```python
from build123d import *

# Parameters (mm, degrees)
F0_R     = 2.0574
F1_DEPTH = 12.7


# Not quite as in the source:
# - a feature names something its author has since deleted; it is built from what else it names


with BuildPart() as f1:
    # F0 (on Top) → F1 (new body)
    with BuildSketch(Plane.XY):
        with BuildLine():
            Line((0, 8.9704120984), (0, -13.0232248562))
            Line((0, -13.0232248562), (26.7917899333, -13.0232248562))
            ThreePointArc((26.7917899333, -13.0232248562), (29.7688, -0.5781617802), (32.7458100667, -13.0232248562))
            Line((32.7458100667, -13.0232248562), (59.5376, -13.0232248562))
            Line((59.5376, -13.0232248562), (59.5376, 8.9704120984))
            Line((59.5376, 8.9704120984), (0, 8.9704120984))
        make_face()
        with Locations((8.1026, -5.2786845261)):
            Circle(F0_R, mode=Mode.SUBTRACT)
        with Locations((51.435, -5.2786845261)):
            Circle(F0_R, mode=Mode.SUBTRACT)
    extrude(amount=F1_DEPTH)


solid = f1.part
```
Check sheet for the modelled part. Datum: model origin and axes. Units: mm. Round coordinates to 2 decimals unless told otherwise and drop trailing zeros. Loops run counter-clockwise (first coordinate to the right, second up) from the corner with the lowest first, then second, coordinate; pieces in that order, holes last. Notation, with made-up numbers: (89, -13.5) - (126, -13.5) arc R12 ccw to (126, 1.5) - close; hole circle Ø7 at (1, -24). An arc over 180 degrees is marked (long way). Write item = value, one per line. Start each with the question number.
Q1. Depth check by flat-ended pin: P1, Ø3.5, axis at x = 8.1, y = -5.28, coming from the -Z side; P2, Ø2, axis at x = 10, y = 0, coming from the -Z side. Enter the tip coordinate at first touch or a pass-through.
Q2. Section check B-B (z = 4). Record the boundary of the cut face in (x, y) (3 decimals), plus the area to 3 significant figures.
Q3. Section check A-A (y = -8.75). Record the boundary of the cut face in (x, z), plus the area to 3 significant figures.
Q4. Section check C-C (y = -4.25). Record the boundary of the cut face in (x, z).
Q5. Release check for a two-part mould opening along X. For faces 1 (the face through (30, 8.97, 6)), 2 (the face through (0, -2, 6)), 3 (the face through (53.397, -4.661, 6.261)) record: pulls with the +X half, pulls with the -X half, needs draft (parallel to the pull), parting line crosses it, or undercut.
Q6. Thickness scan on L1, parallel to X at y = -3.5, z = 10.5; L2, parallel to X at y = -7.5, z = 4.25; L3, parallel to Y at x = 26, z = 11. Record the ranges inside material, lowest first.
Derived:
q1.P1 = through
q1.P2 = 0
q2.outline = (0, -13.023) - (26.792, -13.023) arc R6.579 cw (long way) to (32.746, -13.023) - (59.538, -13.023) - (59.538, 8.97) - (0, 8.97) - close; hole circle Ø4.115 at (8.103, -5.279); hole circle Ø4.115 at (51.435, -5.279)
q2.area = 1,150 mm^2
q3.outline = (0, 0) - (23.39, 0) - (23.39, 12.7) - (0, 12.7) - close; (36.15, 0) - (59.54, 0) - (59.54, 12.7) - (36.15, 12.7) - close
q3.area = 594 mm^2
q4.outline = (0, 0) - (6.32, 0) - (6.32, 12.7) - (0, 12.7) - close; (9.88, 0) - (23.87, 0) - (23.87, 12.7) - (9.88, 12.7) - close; (35.67, 0) - (49.65, 0) - (49.65, 12.7) - (35.67, 12.7) - close; (53.22, 0) - (59.54, 0) - (59.54, 12.7) - (53.22, 12.7) - close
q5.face_1 = needs draft
q5.face_2 = pulls with the -X half
q5.face_3 = undercut
q6.L1 = 0 to 7.07, 9.14 to 24.3, 35.24 to 50.4, 52.47 to 59.54
q6.L2 = 0 to 23.2, 36.34 to 59.54
q6.L3 = -13.02 to -12.55, -1.76 to 8.97
